Autodesk Inventor part; units mm, degrees
ref_plane "YZ Plane" through (0, 0, 0) normal (1, 0, 0) x (0, 1, 0)
ref_plane "XZ Plane" through (0, 0, 0) normal (0, 1, 0) x (-1, 0, 0)
ref_plane "XY Plane" through (0, 0, 0) normal (0, 0, 1) x (1, 0, 0)
sketch "Sketch1" plane through (0, 0, 0) normal (0, 1, 0) x (-1, 0, 0)
  line L0 (8, 10) -> (-8, 10)
  line L1 (-10, 8) -> (-10, -8)
  line L2 (-8, -10) -> (8, -10)
  line L3 (10, -8) -> (10, 8)
  line L4 (10, 10) -> (-10, -10) construction
  line L5 (-10, 10) -> (10, -10) construction
  line L6 (8, 8) -> (-8, 8)
  line L7 (-8, 8) -> (-8, -8)
  line L8 (-8, -8) -> (8, -8)
  line L9 (8, -8) -> (8, 8)
  arc A0 (10, 8) -> (8, 10) centre (8, 8) ccw
  arc A1 (8, -10) -> (10, -8) centre (8, -8) ccw
  arc A2 (-10, -8) -> (-8, -10) centre (-8, -8) ccw
  arc A3 (-8, 10) -> (-10, 8) centre (-8, 8) ccw
  point P0 (0, 0)
  dimension "d0" = 20
  dimension "d1" = 20
  dimension "d2" = 2
  dimension "d3" = 2
  dimension "d4" = 2
extrude "Extrusion1" add sketch "Sketch1" along normal blind 144
sketch "Sketch2" plane through (10, 0, 8) normal (1, 0, 0) x (0, 0, -1)
  line L0 (0, 0) -> (16, 0)
  line L1 (16, 0) -> (16, 144)
  point P0 (8, 0)
  point P1 (8, 8)
  point P2 (8, 0)
  point P3 (8, 16)
  point P4 (8, 24)
  point P5 (8, 32)
  dimension "d7" = 8
  dimension "d10" = 8
hole "Hole1" at (10, 8, 0) at (10, 16, 0) at (10, 24, 0) at (10, 32, 0) direction (-1, 0, 0) diameter 4.05 end through all
sketch "Sketch3" plane through (-8, 0, 10) normal (0, 0, 1) x (1, 0, 0)
  line L0 (0, 144) -> (16, 144)
  line L1 (0, 0) -> (0, 144)
  point P0 (8, 0)
  point P1 (8, 135)
  point P2 (8, 144)
  dimension "d22" = 9
  dimension "d23" = 8
hole "Hole2" at (0, 135, 10) direction (0, 0, -1) diameter 2.45 depth 2
properties part number "suspension2chassisarm"
Geometry: final body of the model. Coordinates: model frame, mm. A direction names the side the tool comes from. Round coordinates to 2 decimals unless told otherwise and drop trailing zeros. Loops run counter-clockwise (first coordinate to the right, second up) from the corner with the lowest first, then second, coordinate; pieces in that order, holes last. Notation, with made-up numbers: (44.5, 53.5) -> (94.5, 53.5) arc R17 ccw to (94.5, 63.5) -> close; hole circle Ø10 at (48, 11). An arc over 180 degrees is marked (long way). Write each question's results on one line, items separated by ' | '.
Item 1: Set-up query: faces 1 (the face through (-0.054, 136.224, 8.986)), 2 (the face through (0, 71, 8)), 3 (the face through (9, 0, 0)). Return all of +Z, -Z, +X, -X, +Y, -Y with unobstructed straight access to the full face (end or side cutting, diameter ignored); none if empty.
Answers below:
face 1: +Z | face 2: +Y, -Y | face 3: +Z, -Z, +X, -X, -Y
Item 2: Cut plane A-A on y = 8. Return the cut outline in (x, z) (3 decimals).
Answers below:
outline: (-10, -8) arc R2 ccw to (-8, -10) -> (8, -10) arc R2 ccw to (10, -8) -> (10, -2.025) -> (8, -2.025) -> (8, -8) -> (-8, -8) -> (-8, -2.025) -> (-10, -2.025) -> close; (-10, 2.025) -> (-8, 2.025) -> (-8, 8) -> (8, 8) -> (8, 2.025) -> (10, 2.025) -> (10, 8) arc R2 ccw to (8, 10) -> (-8, 10) arc R2 ccw to (-10, 8) -> close
Item 3: Cut plane B-B on z = -6. Return the cut outline in (x, y), and give its area (3 significant figures).
Answers below:
outline: (-10, 0) -> (-8, 0) -> (-8, 144) -> (-10, 144) -> close; (8, 0) -> (10, 0) -> (10, 144) -> (8, 144) -> close | area: 576 mm²
Item 4: Cut plane D-D on y = 61. Return the cut outline in (x, z), and give its area (3 significant figures).
Answers below:
outline: (-10, -8) arc R2 ccw to (-8, -10) -> (8, -10) arc R2 ccw to (10, -8) -> (10, 8) arc R2 ccw to (8, 10) -> (-8, 10) arc R2 ccw to (-10, 8) -> close; hole (-8, -8) -> (8, -8) -> (8, 8) -> (-8, 8) -> close | area: 141 mm²
Item 5: Line query: probe 1 along Y at (x, z) = (9.4, 0) (3 decimals); probe 2 along Y at (x, z) = (0, 9.4) (3 decimals); probe 3 along Z at (x, y) = (7.25, 12). Output: solid intervals per line, ascending. Write a range as [from, to].
Answers below:
probe 1: y = [0, 5.975], [10.025, 13.975], [18.025, 21.975], [26.025, 29.975], [34.025, 144] | probe 2: y = [0, 133.775], [136.225, 144] | probe 3: z = [-10, -8], [8, 10]
Item 6: Cut plane C-C on x = -5.5. Return the cut outline in (y, z).
Answers below:
outline: (0, -10) -> (144, -10) -> (144, -8) -> (0, -8) -> close; (0, 8) -> (144, 8) -> (144, 10) -> (0, 10) -> close
Item 7: Pin query (flat end, axial travel): pin 1 Ø5.5 at (y, z) = (16, 0) entering from +X; pin 2 Ø3.5 at (y, z) = (8, 0) entering from -X. Return the tip coordinate at first contact, or that it passes through.
Answers below:
pin 1: stops at x = 10 | pin 2: passes through
Item 8: Pull-direction query (X, two-part tool) for faces 4 (the face through (-9.01, 29.99, 0.26)), 5 (the face through (-10, 71, 0)), 6 (the face through (8, 71, 0)); classes: pulls with the +X half, pulls with the -X half, needs draft (parallel to the pull), parting line crosses it, or undercut.
Answers below:
face 4: needs draft | face 5: pulls with the -X half | face 6: undercut
